Can you work these out from the drawing? Everything is in mm from the part's minimum corner. Coordinates: 2 decimals unless noted, no trailing zeros. Order: outer loops, then holes, each group sorted by start corner. A loop starts at its lowest first (then second) coordinate and runs counter-clockwise, first axis right, second up. Notation, with made-up numbers: (47.5, 48.5) -> (105.5, 48.5) arc R35 cw to (105.5, 86.5) -> close; hole circle Ø8 at (60, 13). An arc over 180 degrees is marked (long way). Use a Markdown table: item, result. Add a question column.
1) If we section it at A-A (y = 3): Give the number of separate pieces and of enclosed holes in the cut face, plus the area to 3 significant figures.
2) If we section it at C-C (z = 32.5): Write out the boundary of the cut face in (x, y).
3) Will these pins go through, and if not, where does the flat tip stop? pin 1 Ø1.2 at (x, z) = (53.5, 2.5) entering from +Y; pin 2 Ø0.8 at (y, z) = (4.5, 65.5) entering from -X; pin 3 Ø0.5 at (x, y) = (8, 4) entering from -Z.
4) If I drill on L1, parallel to Z at x = 8, y = 3.3; L2, parallel to Z at x = 53.5, y = 3.45; L3, parallel to X at y = 3.9, z = 2.5, over which ranges is the centre line in solid material (lowest first)? Write a range as [from, to].
5) If we section it at B-B (x = 42): Write out the boundary of the cut face in (y, z).
6) Thinking about a two-plate mould opening in Z: for the marked faces 1 and 2, which applies, +Z half, -Z half, draft (parallel to the pull), parting line (faces both ways), or undercut?
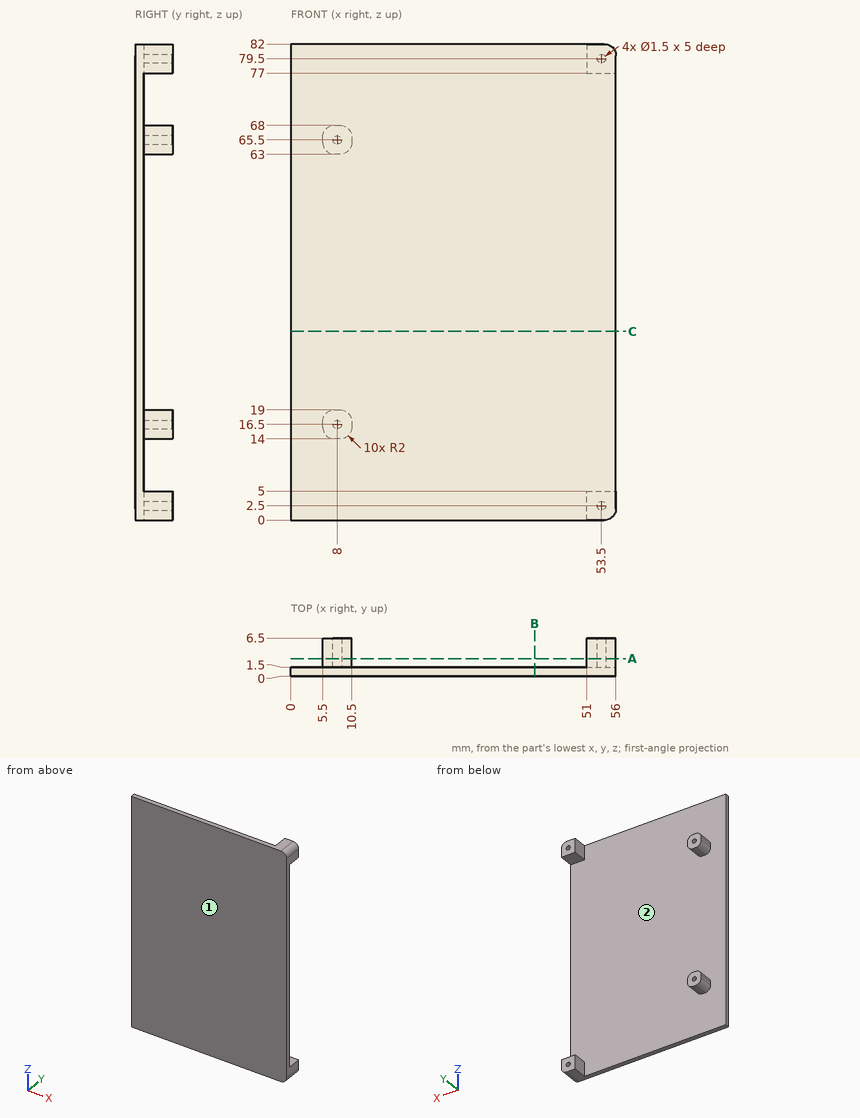
Answer sheet:
| question | item | result |
|---|---|---|
| 1 | separate pieces | 4 |
| 1 | enclosed holes | 4 |
| 1 | area | 84.3 mm2 |
| 2 | outline | (0, 0) -> (56, 0) -> (56, 1.5) -> (0, 1.5) -> close |
| 3 | pin 1 | y = 1.5 |
| 3 | pin 2 | x = 5.5 |
| 3 | pin 3 | z = 14 |
| 4 | L1 | [14, 15.75], [17.25, 19], [63, 64.75], [66.25, 68] |
| 4 | L2 | [0, 1.75], [3.25, 5], [77, 78.75], [80.25, 82] |
| 4 | L3 | [51, 52.75], [54.25, 56] |
| 5 | outline | (0, 0) -> (1.5, 0) -> (1.5, 82) -> (0, 82) -> close |
| 6 | face 1 | draft |
| 6 | face 2 | undercut |
